For this review, use the dimensioned drawing (mm, ordinates from the lowest corner) and the shaded views. A direction names the side the tool comes from. Give positions to 0.01 mm unless a question says otherwise; leave off trailing zeros. Write each loop counter-clockwise with the first axis right and the second up, starting at its lowest first coordinate (ties: lowest second). Pieces come first, ordered by that corner, then holes. Notation, with made-up numbers: (81.25, 81.5) - (113.25, 81.5) arc R22 ccw to (113.25, 105.5) - close; hole circle Ø1 at (-10, 41). An arc over 180 degrees is marked (long way). Use a Markdown table: item, result. Add a question column.
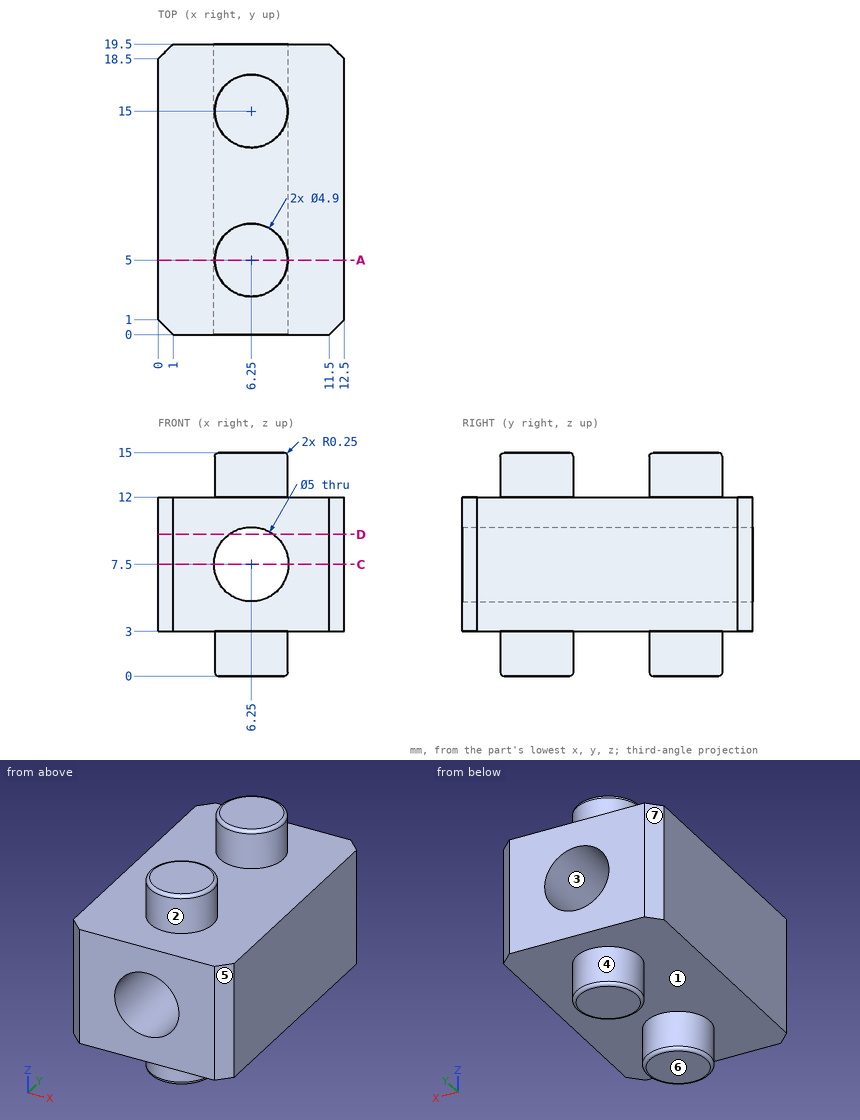
(1) Mouldability with a two-part tool opening along Y and no side actions: class the marked faces 4, 5, 6 and 7 as +Y half, -Y half, draft (parallel to the pull), parting line (faces both ways), or undercut.
(2) Add section D-D (z = 9.5). State the section outline as (x, y) points, and give its area (3 significant figures).
(3) Add section A-A (y = 5). State the section outline as (x, z) points.
(4) Add section C-C (z = 7.5). State the section outline as (x, y) points.
(5) Insertion check: pin 1 (6 mm diameter, centred on x = 6.25, z = 7.5, fed in from +Y); pin 2 (2 mm diameter, centred on x = 4.5, y = 9, fed in from +Z). Each pin has a flat end and moves straight along its axis. Give the tip position at first contact, or say it passes through.
(6) Tool access review of the marked faces 1, 2 and 3: name each direction out of +Z, -Z, +X, -X, +Y, -Y from which nothing blocks a thin tool from reaching the whole face with its end or side.
(7) For line 1 along Y through (x, z) = (6.25, 14.5); line 2 along Z through (x, y) = (11, 16.5); line 3 along X through (y, z) = (13.5, 7.5), list the stretches that pass through material, from the lowest coordinate up.
Answers follow:
| question | item | result |
|---|---|---|
| 1 | face 4 | undercut |
| 1 | face 5 | -Y half |
| 1 | face 6 | draft |
| 1 | face 7 | +Y half |
| 2 | outline | (0, 1) - (1, 0) - (4.75, 0) - (4.75, 19.5) - (1, 19.5) - (0, 18.5) - close; (7.75, 0) - (11.5, 0) - (12.5, 1) - (12.5, 18.5) - (11.5, 19.5) - (7.75, 19.5) - close |
| 2 | area | 183 mm^2 |
| 3 | outline | (0, 3) - (3.8, 3) - (3.8, 0.25) arc R0.25 ccw to (4.05, 0) - (8.45, 0) arc R0.25 ccw to (8.7, 0.25) - (8.7, 3) - (12.5, 3) - (12.5, 12) - (8.7, 12) - (8.7, 14.75) arc R0.25 ccw to (8.45, 15) - (4.05, 15) arc R0.25 ccw to (3.8, 14.75) - (3.8, 12) - (0, 12) - close; hole circle Ø5 at (6.25, 7.5) |
| 4 | outline | (0, 1) - (1, 0) - (3.75, 0) - (3.75, 19.5) - (1, 19.5) - (0, 18.5) - close; (8.75, 0) - (11.5, 0) - (12.5, 1) - (12.5, 18.5) - (11.5, 19.5) - (8.75, 19.5) - close |
| 5 | pin 1 | y = 19.5 |
| 5 | pin 2 | z = 12 |
| 6 | face 1 | -Z |
| 6 | face 2 | +Z |
| 6 | face 3 | +Y, -Y |
| 7 | line 1 | 2.55 to 7.45, 12.55 to 17.45 |
| 7 | line 2 | 3 to 12 |
| 7 | line 3 | 0 to 3.75, 8.75 to 12.5 |
